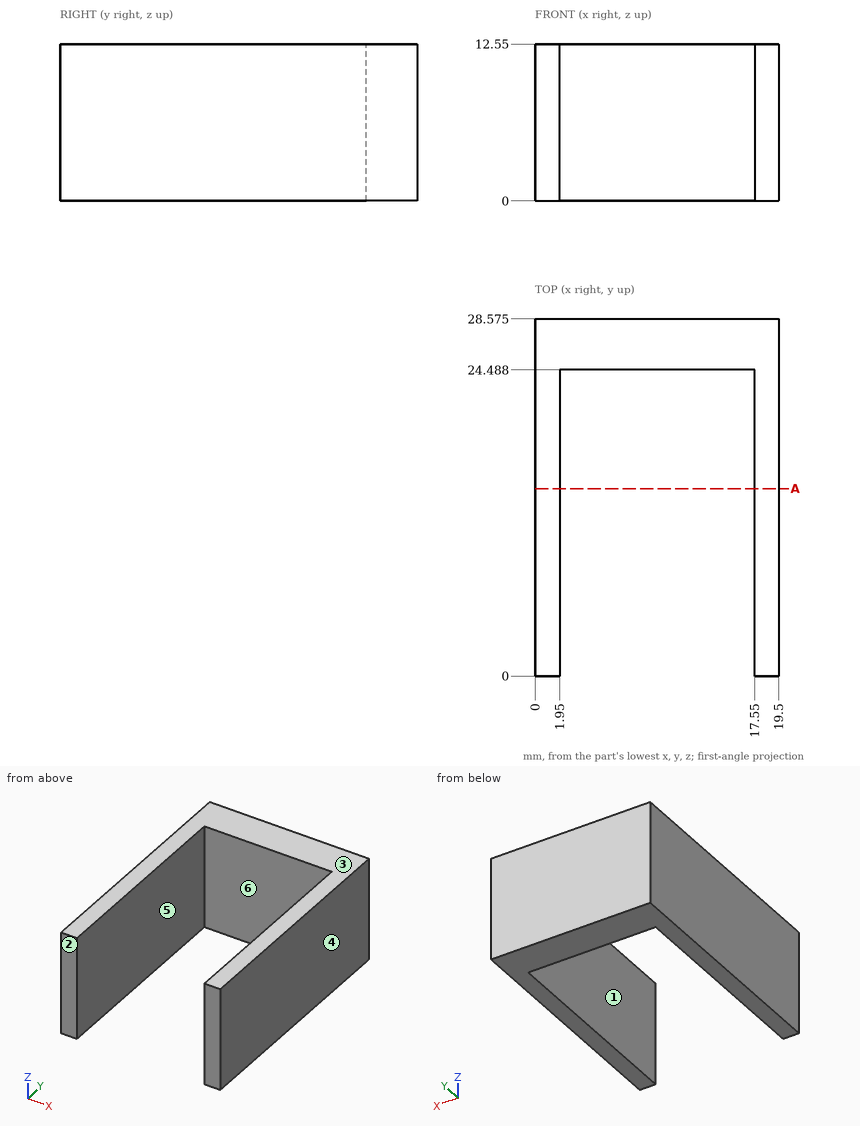
Geometry check sheet. Reference: drawing and pictorial views, mm from the part's lowest x, y, z. A direction names the side the tool comes from. Give positions to 0.01 mm unless a question says otherwise; leave off trailing zeros. Order: outer loops, then holes, each group sorted by start corner. A loop starts at its lowest first (then second) coordinate and runs counter-clockwise, first axis right, second up. Notation, with made-up numbers: (-40, -10.75) -> (-4, -10.75) arc R22 cw to (-4, 17.25) -> close; hole circle Ø2 at (25.5, 45). An arc over 180 degrees is marked (long way). Write each question's results on one line, items separated by ' | '. Start each with the question number.
(1) Mould release check, pull along X, two halves, no side actions. Record for the marked faces 3, 4, 5 and 6: pulls with the +X half, pulls with the -X half, needs draft (parallel to the pull), parting line crosses it, or undercut.
(2) Sectioned sample at A-A (y = 15). Enter the section's corners in (x, z).
(3) Scan lines: line 1 (X direction, y = 2.5, z = 11.75); line 2 (Y direction, x = 15.75, z = 3.25) (1 decimal). Record each from-to range of solid material in increasing order.
(4) Access from +Z, -Z, +X, -X, +Y, -Y to the whole of each face (thin tool, end or side, straight path). Record for the marked faces 1 and 2.
(5) Gauge pin test, flat ends, axial feed: P1, Ø1, axis at y = 25.5, z = 3.5, coming from the -X side; P2, Ø5, axis at x = 13.5, y = 18, coming from the +Z side; P3, Ø6, axis at x = 11.5, z = 7, coming from the -Y side. Record the tip position at first contact, or that the pin passes through.
Answer below:
1) face 3: needs draft | face 4: pulls with the +X half | face 5: undercut | face 6: undercut
2) outline: (0, 0) -> (1.95, 0) -> (1.95, 12.55) -> (0, 12.55) -> close; (17.55, 0) -> (19.5, 0) -> (19.5, 12.55) -> (17.55, 12.55) -> close
3) line 1: 0 to 1.95, 17.55 to 19.5 | line 2: 24.5 to 28.6
4) face 1: +Z, -Z, -Y | face 2: +Z, -Z, +X, -X, -Y
5) P1: x = 0 | P2: through | P3: y = 24.49
